Read the model definition and answer for the solid it produces. Units are mm, in the model's axes. Coordinates: 2 decimals unless noted, no trailing zeros. Order: outer loops, then holes, each group sorted by start corner. A loop starts at its lowest first (then second) coordinate and runs counter-clockwise, first axis right, second up. Notation, with made-up numbers: (19, -13.5) -> (29, -13.5) arc R22 cw to (29, 0.5) -> close; hole circle Ø2 at (4.25, -21.5). An arc over 180 degrees is marked (long way). Return JSON: item names as keys, results as strings. Group by question number.
```python
from build123d import *

# Parameters (mm, degrees)
F0_W     = 1092.2
F0_H     = 660.4
F0_W_2   = 762
F0_H_2   = 381
F0_W_3   = 736.6
F0_H_3   = 355.6
F1_DEPTH = 6.35
F2_DEPTH = 12.7


with BuildPart() as f1:
    # F0 (on Top) → F1 (new body)
    with BuildSketch(Plane.XY):
        with Locations((-500.782648, 283.866385)):
            Rectangle(F0_W, F0_H)
        with Locations((-500.782648, 283.866385)):
            Rectangle(F0_W_2, F0_H_2, mode=Mode.SUBTRACT)
        with Locations((-500.782648, 283.866385)):
            Rectangle(F0_W_2, F0_H_2)
        with Locations((-500.782648, 283.866385)):
            Rectangle(F0_W_3, F0_H_3, mode=Mode.SUBTRACT)
    extrude(amount=F1_DEPTH)

    # F0 (on Top) → F2 (join)
    with BuildSketch(Plane.XY):
        with Locations((-500.782648, 283.866385)):
            Rectangle(F0_W, F0_H)
        with Locations((-500.782648, 283.866385)):
            Rectangle(F0_W_2, F0_H_2, mode=Mode.SUBTRACT)
    extrude(amount=F2_DEPTH)


solid = f1.part
```
1. Find section B-B on z = 3. Determine the outline of the cut face in (x, y), and give its area (3 significant figures).
2. Given pin 1 (5 mm diameter, centred on x = -881, y = 297, fed in from -Z), flat-ended and moving along its own axis, determine where the tip first touches the part or whether it passes through.
3. Straight lines are drawn through the part: L1, parallel to X at y = 327, z = 2.25; L2, parallel to Y at x = -554.5, z = 4; L3, parallel to Y at x = -403, z = 9. For each, find the intervals that lie inside material, in ascending order.
4. For a pull along Y with two mould halves and no side action, classify faces 1 (the face through (-615, 101, 6.35)), 2 (the face through (-508, 509, 0)) as released by +Y, released by -Y, zero draft, split by the parting line, or undercut.
5. Find section C-C on y = 402.5. Determine the outline of the cut face in (x, z).
6. Find section A-A on x = -258. Determine the outline of the cut face in (y, z).
Result:
{
 "1": {"outline": "(-1046.88, -46.33) -> (45.32, -46.33) -> (45.32, 614.07) -> (-1046.88, 614.07) -> close; hole (-869.08, 106.07) -> (-132.48, 106.07) -> (-132.48, 461.67) -> (-869.08, 461.67) -> close", "area": "459,000 mm^2"},
 "2": {"pin 1": "z = 0"},
 "3": {"L1": "-1046.88 to -869.08, -132.48 to 45.32", "L2": "-46.33 to 106.07, 461.67 to 614.07", "L3": "-46.33 to 93.37, 474.37 to 614.07"},
 "4": {"face 1": "undercut", "face 2": "zero draft"},
 "5": {"outline": "(-1046.88, 0) -> (-869.08, 0) -> (-869.08, 6.35) -> (-881.78, 6.35) -> (-881.78, 12.7) -> (-1046.88, 12.7) -> close; (-132.48, 0) -> (45.32, 0) -> (45.32, 12.7) -> (-119.78, 12.7) -> (-119.78, 6.35) -> (-132.48, 6.35) -> close"},
 "6": {"outline": "(-46.33, 0) -> (106.07, 0) -> (106.07, 6.35) -> (93.37, 6.35) -> (93.37, 12.7) -> (-46.33, 12.7) -> close; (461.67, 0) -> (614.07, 0) -> (614.07, 12.7) -> (474.37, 12.7) -> (474.37, 6.35) -> (461.67, 6.35) -> close"}
}
